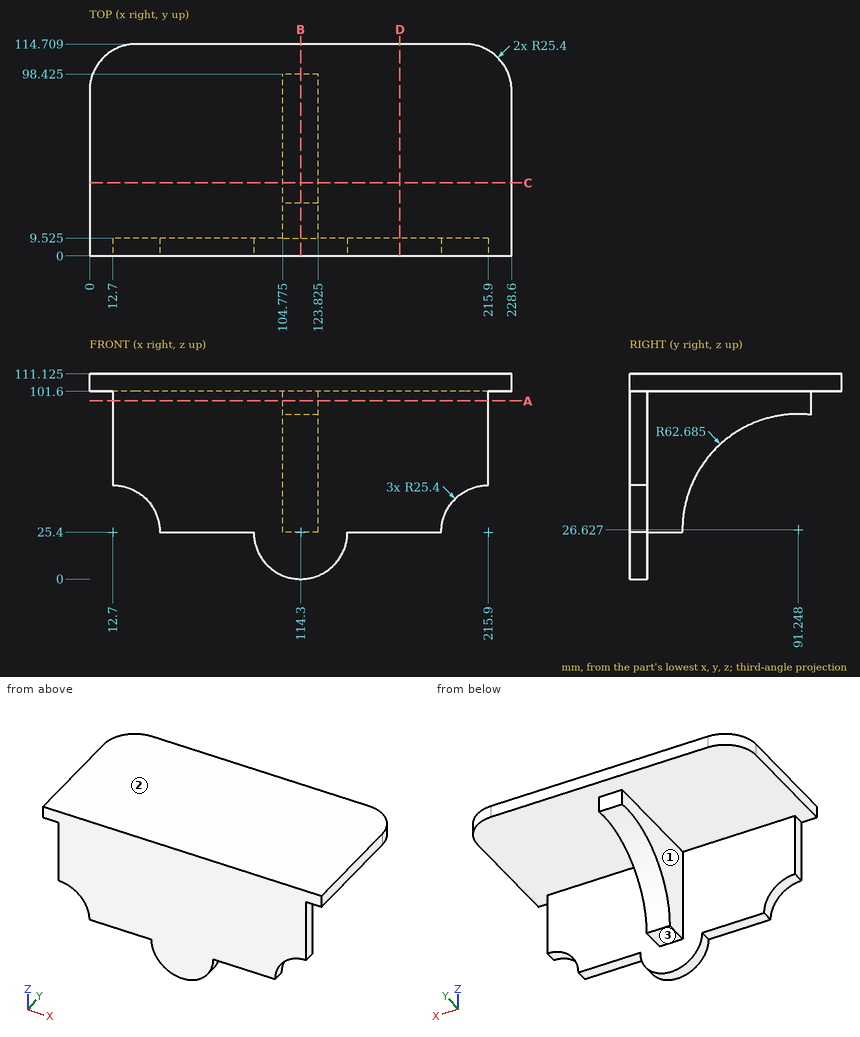
Study the drawing (mm; zero at the part's minimum x, y, z) and answer. A direction names the side the tool comes from. Round coordinates to 2 decimals unless told otherwise and drop trailing zeros. Loops run counter-clockwise (first coordinate to the right, second up) from the corner with the lowest first, then second, coordinate; pieces in that order, holes last. Notation, with made-up numbers: (70, 67) - (81, 67) arc R29 ccw to (81, 100) - close; hole circle Ø10 at (-28.75, 27.5). An arc over 180 degrees is marked (long way). Use one line per item in the form item = value. Start each with the question number.
1. Consider line 1 (X direction, y = 97, z = 100) (1 decimal); line 2 (Z direction, x = 183, y = 43) (1 decimal); line 3 (Y direction, x = 129, z = 37) (1 decimal). Determine where each line is inside the solid, lowest interval first. Write a range as [from, to].
2. The part is cut by section C-C on y = 39.5. Determine the outline of the cut face in (x, z) (1 decimal), then the cut area to 3 significant figures.
3. The part is cut by section D-D on x = 168. Determine the outline of the cut face in (y, z) (1 decimal), then the cut area to 3 significant figures.
4. Given pin 1 Ø5 at (y, z) = (7, 85) entering from +X; pin 2 Ø1 at (x, y) = (81.5, 12) entering from -Z; pin 3 Ø5 at (x, z) = (196, 76.5) entering from +Y (3 decimals), each flat-ended and moving along its own axis, determine where each tip first touches the part or whether it passes through.
5. The part is cut by section B-B on x = 114.3. Determine the outline of the cut face in (y, z) (1 decimal), then the cut area to 3 significant figures.
6. The part is cut by section A-A on z = 96.5. Determine the outline of the cut face in (x, y) (1 decimal).
7. A tool of negligible diameter and unlimited length cuts with its end or side. For the marked faces 1, 2 and 3, from which of +Z, -Z, +X, -X, +Y, -Y can it reach the whole face along a straight path? Write none if from no direction.
Geometry check:
q1.line_1 = [104.8, 123.8]
q1.line_2 = [101.6, 111.1]
q1.line_3 = [0, 9.5]
q2.outline = (0, 101.6) - (104.8, 101.6) - (104.8, 62) - (123.8, 62) - (123.8, 101.6) - (228.6, 101.6) - (228.6, 111.1) - (0, 111.1) - close
q2.area = 2,930 mm^2
q3.outline = (0, 25.4) - (9.5, 25.4) - (9.5, 101.6) - (114.7, 101.6) - (114.7, 111.1) - (0, 111.1) - close
q3.area = 1,820 mm^2
q4.pin_1 = 215.9
q4.pin_2 = 101.6
q4.pin_3 = 9.525
q5.outline = (0, 0) - (9.5, 0) - (9.5, 25.4) - (28.6, 25.4) arc R62.7 cw to (98.4, 88.9) - (98.4, 101.6) - (114.7, 101.6) - (114.7, 111.1) - (0, 111.1) - close
q5.area = 5,210 mm^2
q6.outline = (12.7, 0) - (215.9, 0) - (215.9, 9.5) - (123.8, 9.5) - (123.8, 98.4) - (104.8, 98.4) - (104.8, 9.5) - (12.7, 9.5) - close
q7.face_1 = -Z, -X, +Y
q7.face_2 = +Z, +X, -X, +Y, -Y
q7.face_3 = -Z, +X, -X, +Y
